Geometry: see drawing. Coordinates: mm, zero at the bounding-box minimum. A direction names the side the tool comes from. Coordinates: 2 decimals unless noted, no trailing zeros. Order: outer loops, then holes, each group sorted by start corner. A loop starts at its lowest first (then second) coordinate and runs counter-clockwise, first axis right, second up.
Item 1: Mould query, pull axis X, two halves, no side actions, for the marked faces 3 and 4. Classes: released by +X, released by -X, zero draft, split by the parting line, or undercut.
Item 2: Ray query, line 1 (X direction, y = 13, z = 7.75); line 2 (X direction, y = 26, z = 0.75); line 3 (Y direction, x = 13, z = 9). Return the intervals inside material, ascending.
Item 3: Section D-D on x = 80. Return the cut outline in (y, z).
Item 4: Reachability of the marked faces 1 and 2 from +Z, -Z, +X, -X, +Y, -Y: full face, straight path, thin tool, end or side. Return the list, or none.
Item 5: Section C-C on z = 5. State how many separate pieces and enclosed holes the cut face has, then the cut area to 3 significant figures.
Item 6: Section B-B on x = 66.75. Return the cut outline in (y, z), then the cut area to 3 significant figures.
Item 7: Section A-A on y = 20.5. Return the cut outline in (x, z), then the cut area to 3 significant figures.
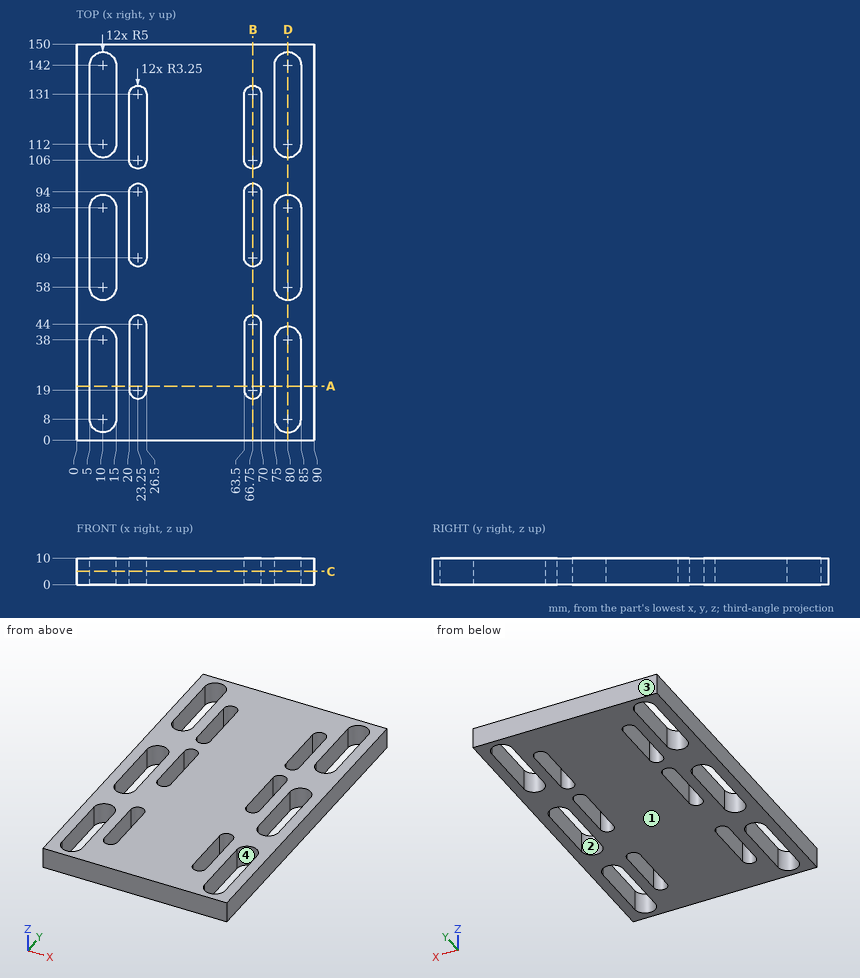
Answer list:
1. face 3: zero draft
1. face 4: undercut
2. line 1: x = 0 to 5, 15 to 75, 85 to 90
2. line 2: x = 0 to 5, 15 to 20, 26.5 to 63.5, 70 to 75, 85 to 90
2. line 3: y = 0 to 4, 42 to 54, 92 to 108, 146 to 150
3. outline: (0, 0) - (3, 0) - (3, 10) - (0, 10) - close; (43, 0) - (53, 0) - (53, 10) - (43, 10) - close; (93, 0) - (107, 0) - (107, 10) - (93, 10) - close; (147, 0) - (150, 0) - (150, 10) - (147, 10) - close
4. face 1: -Z, +X, -X, +Y, -Y
4. face 2: +Z, -Z
5. separate pieces: 1
5. enclosed holes: 12
5. area: 10,100 mm2
6. outline: (0, 0) - (15.75, 0) - (15.75, 10) - (0, 10) - close; (47.25, 0) - (65.75, 0) - (65.75, 10) - (47.25, 10) - close; (97.25, 0) - (102.75, 0) - (102.75, 10) - (97.25, 10) - close; (134.25, 0) - (150, 0) - (150, 10) - (134.25, 10) - close
6. area: 555 mm2
7. outline: (0, 0) - (5, 0) - (5, 10) - (0, 10) - close; (15, 0) - (20, 0) - (20, 10) - (15, 10) - close; (26.5, 0) - (63.5, 0) - (63.5, 10) - (26.5, 10) - close; (70, 0) - (75, 0) - (75, 10) - (70, 10) - close; (85, 0) - (90, 0) - (90, 10) - (85, 10) - close
7. area: 570 mm2
